The model under review builds one solid part; all positions refer to its coordinate system, in mm. A direction names the side the tool comes from. Give positions to 0.01 mm unless a question says otherwise; leave off trailing zeros. Write each loop counter-clockwise with the first axis right and the second up, starting at its lowest first coordinate (ties: lowest second). Pieces come first, ordered by that corner, then holes. Notation, with made-up numbers: M 56,-24.75 L 61,-24.75 A6 cw 61,-16.75 Z; hole C -25,5 d11. An arc over 180 degrees is marked long. Write each question's results on one line, items separated by ' | '. Start each with the question number.
from build123d import *

# Parameters (mm, degrees)
SKETCH_1_W           = 170
SKETCH_1_H           = 170
EXTRUDE_1_DEPTH      = 1.6
SKETCH_2_R           = 1.75
CUT_EXTRUDE_2_DEPTH  = 241.421629643
EXTRUDE_2_DEPTH      = 44.45
EXTRUDE_2_DEPTH_BACK = 3.81
SKETCH_5_W           = 1
SKETCH_5_H           = 158.75


with BuildPart() as part:
    # 草图1 → 凸台-拉伸1 (new body)
    with BuildSketch(Plane.XY):
        with Locations((85, 85)):
            Rectangle(SKETCH_1_W, SKETCH_1_H)
    extrude(amount=EXTRUDE_1_DEPTH)

    # 草图2 → 切除-拉伸2 (cut, through all)
    with BuildSketch(Plane.XY.offset(1.6)):
        with Locations((10.16, 6.35)):
            Circle(SKETCH_2_R)
        with Locations((165.1, 6.35)):
            Circle(SKETCH_2_R)
        with Locations((165.1, 163.83)):
            Circle(SKETCH_2_R)
        with Locations((33.02, 163.83)):
            Circle(SKETCH_2_R)
    extrude(amount=-CUT_EXTRUDE_2_DEPTH, mode=Mode.SUBTRACT)

    # 草图5 → 凸台-拉伸2 (add, two sides: drawn at the far end of the back side and taken through both)
    with BuildSketch(Plane.XY.offset(1.6).offset(-EXTRUDE_2_DEPTH_BACK)):
        with Locations((-0.5, 90.625)):
            Rectangle(SKETCH_5_W, SKETCH_5_H)
    extrude(amount=EXTRUDE_2_DEPTH + EXTRUDE_2_DEPTH_BACK)


solid = part.part
(1) Add section B-B (z = 18.5). State the section outline as (x, y) points, then the cut area to 3 significant figures.
(2) Clearance check with flat-ended pins moving along their axes: P1, Ø22, axis at y = 101, z = 34, coming from the +X side; P2, Ø4, axis at x = 33.02, y = 163.83, coming from the +Z side; P3, Ø4, axis at x = 36, y = 98.5, coming from the -Z side; P4, Ø10, axis at x = 88, z = 3.5, coming from the +Y side. State where each tip first meets the part, or that it passes through.
(3) Machinability: for faces 1 (the flat face through (84, 86, 0)), 2 (the flat face through (84.1, 170, 0.4)), 3 (the flat face through (84, 86, 1.6)), which of the approach directions +Z, -Z, +X, -X, +Y, -Y give a long, thin tool a straight path to every point of the face, cutting with its end or side? Answer none if there is none.
(4) Wall thickness on L1, parallel to X at y = 163.83, z = 0.5; L2, parallel to Y at x = 165.1, z = 1.25; L3, parallel to Y at x = 10.16, z = 0.45: over which ranges is each line inside the solid? List them lowest first.
(5) Add section C-C (x = 46). State the section outline as (y, z) points.
(6) Add section A-A (y = 121). State the section outline as (x, z) points, then the cut area to 3 significant figures.
Calculated:
1) outline: M -1,11.25 L 0,11.25 L 0,170 L -1,170 Z | area: 159 mm²
2) P1: stops at x = 0 | P2: stops at z = 1.6 | P3: stops at z = 0 | P4: stops at y = 170
3) face 1: -Z, +X, +Y, -Y | face 2: +Z, -Z, +X, -X, +Y | face 3: +Z, +X, +Y, -Y
4) L1: x = -1 to 31.27, 34.77 to 163.35, 166.85 to 170 | L2: y = 0 to 4.6, 8.1 to 162.08, 165.58 to 170 | L3: y = 0 to 4.6, 8.1 to 170
5) outline: M 0,0 L 170,0 L 170,1.6 L 0,1.6 Z
6) outline: M -1,-2.21 L 0,-2.21 L 0,0 L 170,0 L 170,1.6 L 0,1.6 L 0,46.05 L -1,46.05 Z | area: 320 mm²
